```python
from build123d import *

# Parameters (mm, degrees)
F0_W     = 76.2
F0_H     = 50.8
F1_DEPTH = 50.8
F3_DEPTH = 76.201


with BuildPart() as f1:
    # F0 (on Front) → F1 (new body)
    with BuildSketch(Plane.XZ):
        with Locations((38.1, 25.4)):
            Rectangle(F0_W, F0_H)
    extrude(amount=F1_DEPTH)

    # F2 (on face) → F3 (cut, through all)
    with BuildSketch(Plane(origin=(0, 0, 0), x_dir=(0, -1, 0), z_dir=(-1, 0, 0))):
        Polygon((0, 50.8), (0, 25.4), (25.4, 50.8), align=None)
    extrude(amount=-F3_DEPTH, mode=Mode.SUBTRACT)


solid = f1.part
```
The listing builds one solid part. Answer for the finished solid, in the listing's coordinates (mm). Coordinates: 2 decimals unless noted, no trailing zeros. Write each loop counter-clockwise with the first axis right and the second up, starting at its lowest first coordinate (ties: lowest second). Pieces come first, ordered by that corner, then holes. Notation, with made-up numbers: (-27, 72.5) - (-5, 72.5) arc R16 cw to (-5, 80.5) - close; hole circle Ø4 at (-16.75, 65.25). An arc over 180 degrees is marked (long way). Return JSON: item names as keys, results as strings. Group by question number.
1. Given pin 1 (1.5 mm diameter, centred on x = 12.5, z = 31, fed in from +Y); pin 2 (5 mm diameter, centred on x = 52, z = 35, fed in from +Y), each flat-ended and moving along its own axis, determine where each tip first touches the part or whether it passes through.
2. Straight lines are drawn through the part: L1, parallel to Y at x = 57, z = 27; L2, parallel to Y at x = 72, z = 28; L3, parallel to Z at x = 17.5, y = -9.5. For each, find the intervals that lie inside material, in ascending order.
3. A cutting plane is placed at C-C, the plane z = 40. Determine the outline of the cut face in (x, y), plus the area to 3 significant figures.
4. A cutting plane is placed at A-A, the plane x = 15.5. Determine the outline of the cut face in (y, z), plus the area to 3 significant figures.
5. A cutting plane is placed at B-B, the plane y = -8. Determine the outline of the cut face in (x, z).
Ans:
{
 "1": {"pin 1": "y = -4.85", "pin 2": "y = -7.1"},
 "2": {"L1": "-50.8 to -1.6", "L2": "-50.8 to -2.6", "L3": "0 to 34.9"},
 "3": {"outline": "(0, -50.8) - (76.2, -50.8) - (76.2, -14.6) - (0, -14.6) - close", "area": "2,760 mm²"},
 "4": {"outline": "(-50.8, 0) - (0, 0) - (0, 25.4) - (-25.4, 50.8) - (-50.8, 50.8) - close", "area": "2,260 mm²"},
 "5": {"outline": "(0, 0) - (76.2, 0) - (76.2, 33.4) - (0, 33.4) - close"}
}
